```python
from build123d import *

# Parameters (mm, degrees)
F0_R     = 1.25
F0_W     = 30
F0_H     = 2
F1_DEPTH = 3
F2_DEPTH = 3
F3_DEPTH = 2


with BuildPart() as f1:
    # F0 (on Top) → F1 (new body)
    with BuildSketch(Plane.XY):
        Polygon((-5.94798, -6.372835), (-7.07298, -6.372835), (-7.07298, -8.372835), (-7.07298, -13.872835), (-2.82298, -13.872835), (-2.82298, -8.372835), (-2.82298, -6.372835), (-3.94798, -6.372835), align=None)
        with Locations((-4.94798, -11.747835)):
            Circle(F0_R, mode=Mode.SUBTRACT)
        with Locations((-4.94798, -8.497835)):
            Circle(F0_R, mode=Mode.SUBTRACT)
        with Locations((-22.07298, -7.372835)):
            Rectangle(F0_W, F0_H)
        with BuildLine():
            Line((-5.94798, 10.273063), (-5.94798, -6.372835))
            Line((-5.94798, -6.372835), (-3.94798, -6.372835))
            Line((-3.94798, -6.372835), (-3.94798, 10.273063))
            ThreePointArc((-3.94798, 10.273063), (-4.94798, 10.127165), (-5.94798, 10.273063))
        make_face()
        with BuildLine():
            ThreePointArc((-1.44798, 13.627165), (-7.03963, 16.433408), (-5.94798, 10.273063))
            Line((-5.94798, 10.273063), (-5.94798, 11.895114))
            ThreePointArc((-5.94798, 11.895114), (-5.94798, 15.359216), (-2.94798, 13.627165))
            ThreePointArc((-2.94798, 13.627165), (-3.215929, 12.627165), (-3.94798, 11.895114))
            Line((-3.94798, 11.895114), (-3.94798, 10.273063))
            ThreePointArc((-3.94798, 10.273063), (-2.141737, 11.535515), (-1.44798, 13.627165))
        make_face()
        with Locations((12.17702, -7.372835)):
            Rectangle(F0_W, F0_H)
        with BuildLine():
            Line((-5.94798, 11.895114), (-5.94798, 10.273063))
            ThreePointArc((-5.94798, 10.273063), (-4.94798, 10.127165), (-3.94798, 10.273063))
            Line((-3.94798, 10.273063), (-3.94798, 11.895114))
            ThreePointArc((-3.94798, 11.895114), (-4.94798, 11.627165), (-5.94798, 11.895114))
        make_face()
        with Locations((-4.94798, -8.497835)):
            Circle(F0_R)
        with Locations((-4.94798, -11.747835)):
            Circle(F0_R)
    extrude(amount=-F1_DEPTH)

    # F0 (on Top) → F2 (join)
    with BuildSketch(Plane.XY):
        Polygon((-5.94798, -6.372835), (-7.07298, -6.372835), (-7.07298, -8.372835), (-7.07298, -13.872835), (-2.82298, -13.872835), (-2.82298, -8.372835), (-2.82298, -6.372835), (-3.94798, -6.372835), align=None)
        with Locations((-4.94798, -11.747835)):
            Circle(F0_R, mode=Mode.SUBTRACT)
        with Locations((-4.94798, -8.497835)):
            Circle(F0_R, mode=Mode.SUBTRACT)
    extrude(amount=F2_DEPTH)

    # F0 (on Top) → F3 (cut)
    with BuildSketch(Plane.XY):
        with Locations((-4.94798, -8.497835)):
            Circle(F0_R)
        with Locations((-4.94798, -11.747835)):
            Circle(F0_R)
    extrude(amount=-F3_DEPTH, mode=Mode.SUBTRACT)


solid = f1.part
```
Build history of the part. All positions in model axes, mm. A direction names the side the tool comes from. Coordinates: 2 decimals unless noted, no trailing zeros. Order: outer loops, then holes, each group sorted by start corner. A loop starts at its lowest first (then second) coordinate and runs counter-clockwise, first axis right, second up.
Item 1: Drill centre lines: L1, parallel to Y at x = -5, z = 1.85; L2, parallel to X at y = -11, z = 1.05; L3, parallel to Y at x = -3.5, z = 0.35. Where is each one in solid material? Low to high.
Filled in:
L1: y = -13.87 to -13, -10.5 to -9.75, -7.25 to -6.37
L2: x = -7.07 to -5.95, -3.95 to -2.82
L3: y = -13.87 to -6.37
Item 2: Drop flat-ended pins along their axis: pin 1 Ø3 at (y, z) = (0.5, -1) entering from -X; pin 2 Ø2 at (x, y) = (-4.95, -11.75) entering from +Z; pin 3 Ø1.8 at (x, z) = (-5, 1) entering from +Y. Give the stop position or say it passes through.
Filled in:
pin 1: stops at x = -5.95
pin 2: stops at z = -2
pin 3: stops at y = -6.37
Item 3: Saw through at A-A on z = 1.75. List the corners of the cut face in (x, y).
Filled in:
outline: (-7.07, -13.87) - (-2.82, -13.87) - (-2.82, -6.37) - (-7.07, -6.37) - close; hole circle Ø2.5 at (-4.95, -11.75); hole circle Ø2.5 at (-4.95, -8.5)
Item 4: Saw through at C-C on y = 3. List the corners of the cut face in (x, z), then the cut area to 3 significant figures.
Filled in:
outline: (-5.95, -3) - (-3.95, -3) - (-3.95, 0) - (-5.95, 0) - close
area: 6.00 mm2
Item 5: Mould opens along Y. For faces 1 (the flat face through (-5.948, 2, -1)), 2 (the flat face through (-22, -8.373, -1)), 3 (the flat face through (-7.073, -10, 0)) say: released by +Y, released by -Y, zero draft, split by the parting line, or undercut.
Filled in:
face 1: undercut
face 2: released by -Y
face 3: zero draft
Item 6: Saw through at B-B on x = -31. List the corners of the cut face in (y, z), then the cut area to 3 significant figures.
Filled in:
outline: (-8.37, -3) - (-6.37, -3) - (-6.37, 0) - (-8.37, 0) - close
area: 6.00 mm2
Item 7: Saw through at D-D on z = -1.3. List the corners of the cut face in (x, y), then the cut area to 3 significant figures.
Filled in:
outline: (-37.07, -8.37) - (-7.07, -8.37) - (-7.07, -13.87) - (-2.82, -13.87) - (-2.82, -8.37) - (27.18, -8.37) - (27.18, -6.37) - (-3.95, -6.37) - (-3.95, 10.27) arc R3.5 ccw (long way) to (-5.95, 10.27) - (-5.95, -6.37) - (-37.07, -6.37) - close; hole circle Ø2.5 at (-4.95, -11.75); hole circle Ø2.5 at (-4.95, -8.5); hole (-5.95, 11.9) arc R2 ccw to (-3.95, 11.9) arc R2 ccw (long way) to start
area: 201 mm2
Item 8: Tool access for faces 4 (the flat face through (-22, -7, 0)), 5 (the cylindrical face through (-3.756, -8.122, 0.465)), 6 (the flat face through (12, -7, 0)), 7 (the flat face through (-3.948, 2, -1)), 8 (the flat face through (12, -8.373, -1)): list every direction of +Z, -Z, +X, -X, +Y, -Y with a clear straight run to the whole face (end or side of a thin tool).
Filled in:
face 4: +Z, -X, +Y, -Y
face 5: +Z
face 6: +Z, +X, +Y, -Y
face 7: +Z, -Z, +X
face 8: +Z, -Z, +X, -Y
